Autodesk Inventor part; units mm, degrees
ref_plane "YZ Plane" through (0, 0, 0) normal (1, 0, 0) x (0, 1, 0)
ref_plane "XZ Plane" through (0, 0, 0) normal (0, 1, 0) x (-1, 0, 0)
ref_plane "XY Plane" through (0, 0, 0) normal (0, 0, 1) x (1, 0, 0)
sketch "Skizze1" plane through (0, 0, 0) normal (0, 0, 1) x (1, 0, 0)
  arc A0 (-7.910725, 24.207043) -> (-7.910891, 20.407043) centre (-6.063513, 22.306962) ccw
  line L0 (-7.910725, 24.207043) -> (-4.216135, 24.206882)
  arc A1 (-4.216301, 20.406882) -> (-4.216135, 24.206882) centre (-6.063513, 22.306962) ccw
  line L1 (-4.216301, 20.406882) -> (-7.910891, 20.407043)
  spline S0 degree 3 poles (4.168227, 35.189684) (1.190462, 36.459804) (-2.249662, 35.164227) (-6.254955, 34.158153) (-11.73606, 32.147863) (-17.267484, 27.437) (-17.397864, 22.280527) (-19.179409, 11.837341) (-24.204265, -4.219772) (-21.912215, -21.361857) (-15.72629, -32.136108) (-8.960071, -34.873142) (-7.734356, -35.206805) knots 0 0 0 0 0.05534958 0.07652777 0.21178189 0.29554676 0.38296386 0.43292215 0.75488434 0.81234043 0.96723776 1 1 1 1
  spline S1 degree 3 poles (-7.734356, -35.206805) (-2.439109, -36.648242) (4.93418, -35.14496) (14.388893, -31.364077) (20.220621, -28.276552) (23.084745, -23.179223) (23.280953, -18.995872) (17.306215, -16.499664) (13.73981, -19.293705) (6.907357, -22.933236) (-1.198572, -27.162074) (-10.305482, -22.9326) (-14.035245, -10.40017) (-9.459871, -0.926027) (-6.833349, 0.315314) (-5.918232, 2.05884) (-5.936684, 4.17913) (-8.288714, 5.230646) (-8.364147, 10.437319) (-1.010592, 14.125066) (4.082108, 20.05073) (3.063503, 26.302613) (2.949283, 28.613576) (3.78883, 29.833993) (5.577793, 31.092404) (6.613193, 32.774527) (5.245759, 34.708646) (4.265654, 35.148112) (4.168227, 35.189684) knots 0 0 0 0 0.1415298 0.17035016 0.24598676 0.2589199 0.29022703 0.32626485 0.37223258 0.38897966 0.48209608 0.50825566 0.62441589 0.64741797 0.71527435 0.72606992 0.74689162 0.80172241 0.81188461 0.84851364 0.9163561 0.94337427 0.94821885 0.96295932 0.96650966 0.98187972 0.99818797 1 1 1 1
  line L2 (-4.216301, 20.406882) -> (-7.910891, 20.407043)
  arc A2 (-4.216301, 20.406882) -> (-4.216135, 24.206882) centre (-6.063513, 22.306962) ccw
  line L3 (-7.910725, 24.207043) -> (-4.216135, 24.206882)
  arc A3 (-7.910725, 24.207043) -> (-7.910891, 20.407043) centre (-6.063513, 22.306962) ccw
  line L4 (-22.994876, 35.829551) -> (22.994876, 35.829551) construction
  line L5 (22.994876, 35.829551) -> (22.994876, -35.829551) construction
  line L6 (22.994876, -35.829551) -> (-22.994876, -35.829551) construction
  line L7 (-22.994876, -35.829551) -> (-22.994876, 35.829551) construction
  line L8 (-22.994876, 35.829551) -> (22.994876, -35.829551) construction
  line L9 (-22.994876, -35.829551) -> (22.994876, 35.829551) construction
  circle A4 centre (3.874552, -36.279551) radius 1.25 construction
  line L10 (1.214575, -35.829551) -> (11.587679, -35.829551) construction
  line L11 (3.874552, -36.279551) -> (3.874552, -35.029551) construction
  circle A5 centre (4.795469, 36.279551) radius 1.25 construction
  line L12 (4.795469, 36.279551) -> (4.795469, 35.029551) construction
  line L13 (3.124047, 35.829551) -> (12.547009, 35.829551) construction
  point P0 (0, 0)
  point P1 (0, 0)
  point P2 (0, 0)
  dimension "d88" = 2.5
  dimension "d91" = 2.5
  dimension "d89" = 0.8
  dimension "d92" = 0.8
sketch "Skizze9" plane through (0, 0, 0) normal (0, 0, 1) x (1, 0, 0)
  line L0 (-30, 46) -> (30, 46)
  line L1 (30, 46) -> (30, -46)
  line L2 (30, -46) -> (-30, -46)
  line L3 (-30, 46) -> (30, -46) construction
  line L4 (30, 46) -> (-30, -46) construction
  spline S0 degree 3 poles (4.168227, 35.189684) (1.190462, 36.459804) (-2.249662, 35.164227) (-6.254955, 34.158153) (-11.73606, 32.147863) (-17.267484, 27.437) (-17.397864, 22.280527) (-19.179409, 11.837341) (-24.204265, -4.219772) (-21.912215, -21.361857) (-15.72629, -32.136108) (-8.960071, -34.873142) (-7.734356, -35.206805) knots 0 0 0 0 0.05534958 0.07652777 0.21178189 0.29554676 0.38296386 0.43292215 0.75488434 0.81234043 0.96723776 1 1 1 1
  spline S1 degree 3 poles (-7.734356, -35.206805) (-2.439109, -36.648242) (4.93418, -35.14496) (14.388893, -31.364077) (20.220621, -28.276552) (23.084745, -23.179223) (23.280953, -18.995872) (17.306215, -16.499664) (13.73981, -19.293705) (6.907357, -22.933236) (-1.198572, -27.162074) (-10.305482, -22.9326) (-14.035245, -10.40017) (-9.459871, -0.926027) (-6.833349, 0.315314) (-5.918232, 2.05884) (-5.936684, 4.17913) (-8.288714, 5.230646) (-8.364147, 10.437319) (-1.010592, 14.125066) (4.082108, 20.05073) (3.063503, 26.302613) (2.949283, 28.613576) (3.78883, 29.833993) (5.577793, 31.092404) (6.613193, 32.774527) (5.245759, 34.708646) (4.265654, 35.148112) (4.168227, 35.189684) knots 0 0 0 0 0.1415298 0.17035016 0.24598676 0.2589199 0.29022703 0.32626485 0.37223258 0.38897966 0.48209608 0.50825566 0.62441589 0.64741797 0.71527435 0.72606992 0.74689162 0.80172241 0.81188461 0.84851364 0.9163561 0.94337427 0.94821885 0.96295932 0.96650966 0.98187972 0.99818797 1 1 1 1
  circle A0 centre (-3.5, -23.6754) radius 2
  circle A1 centre (5.000912, 27.85018) radius 2
  circle A2 centre (-6.3, 8.375362) radius 2
  line L5 (-30, -35.829553) -> (30, -35.829553)
  line L6 (-30, -46) -> (-30, 46)
  line L7 (-30, 35.829552) -> (30, 35.829552)
  point P0 (0, 0)
  point P1 (-2.781906, -35.829553)
  point P2 (1.073951, 35.829552)
  dimension "Laenge_aussen" = 105
  dimension "d68" = 60
  dimension "d69" = 92
  dimension "d180" = 4
  dimension "d182" = 4
  dimension "d183" = 4
  dimension "d184" = 33.5
  dimension "d186" = 24.99909
  dimension "d221" = 36.3
extrude "Extrusion3" add sketch "Skizze9" along normal blind 5 contours L0 L1 L7 L6 | L5 L1 L2 L6
sketch "Skizze11" plane through (0, 0, 0) normal (0, 0, -1) x (-1, 0, 0)
  line L0 (30, -46) -> (-30, -46)
  line L1 (30, 46) -> (30, -46)
  line L2 (-30, -46) -> (30, -46)
  line L3 (30, -46) -> (30, 46)
  line L4 (30, 46) -> (-30, 46)
  line L5 (-30, 46) -> (-30, -46)
  point P0 (0, 0)
extrude "Extrusion4" add sketch "Skizze11" along normal blind 1.5
chamfer "Fasen2" distance 0.5 angle 45 2 edges at (0, -35.8296, 5) (0, 35.8296, 5)
sketch "Skizze15" plane through (-30, 46, 5) normal (0, 1, 0) x (1, 0, 0)
  line L0 (60, 0) -> (0, 0)
  line L1 (0, 6.5) -> (60, 6.5)
  line L2 (60, 0) -> (0, 0)
  line L3 (0, 0) -> (0, 6.5)
  line L4 (0, 6.5) -> (60, 6.5)
  line L5 (60, 6.5) -> (60, 0)
  point P0 (30, 5)
extrude "Extrusion6" add sketch "Skizze15" along normal blind 4
sketch "Skizze16" plane through (-30, -46, 5) normal (0, -1, 0) x (1, 0, 0)
  line L0 (0, -6.5) -> (0, 0)
  line L1 (60, -6.5) -> (0, -6.5)
  line L2 (0, 0) -> (60, 0)
  line L3 (60, 0) -> (60, -6.5)
  line L4 (60, -6.5) -> (0, -6.5)
  line L5 (0, -6.5) -> (0, 0)
  point P0 (30, -5)
extrude "Extrusion7" add sketch "Skizze16" along normal blind 4
sketch "Skizze17" plane through (0, 0, -1.5) normal (0, 0, -1) x (-1, 0, 0)
  line L0 (30, 50) -> (30, -50)
  line L1 (-30, 50) -> (30, 50)
  line L2 (-30, -50) -> (-30, 50)
  line L3 (30, -50) -> (-30, -50)
  point P0 (0, 0)
extrude "Extrusion8" add sketch "Skizze17" along normal blind 3.5
chamfer "Fasen4" distance 0.5 angle 45 2 edges at (0, 50, 5) (0, -50, 5)
sketch "Skizze20" plane through (0, 0, 0) normal (0, 0, 1) x (1, 0, 0)
  line L0 (-30, -50) -> (30, -50)
  line L1 (30, 35.829552) -> (30, -35.829553)
  point P0 (0, 0)
  point P1 (-30, -46.5)
  point P2 (0, 0)
hole "Bohrung10" at (0, 0, 0) direction (0, 0, -1) diameter 5.5 end through all countersink diameter 11.5 countersink angle 90
sketch "Skizze21" plane through (-30, -50, 5) normal (0, -1, 0) x (1, 0, 0)
  line L0 (60, -10) -> (0, -10)
  line L1 (60, 0) -> (0, 0)
  line L2 (60, -0.5) -> (60, -10)
  line L3 (0, -0.5) -> (0, -10)
  point P0 (30, -5)
  point P1 (15, -5)
  point P2 (45, -5)
  point P3 (60, -5.25)
  dimension "d161" = 10
  dimension "d163" = 60
  dimension "d164" = 15
  dimension "d165" = 15
  dimension "d179" = 5
hole "Bohrung11" at (15, -50, 0) at (-15, -50, 0) direction (0, 1, 0) diameter 4.134 depth 6 tip angle 118
chamfer "Fasen5" distance 0.5 angle 45 2 edges at (-15, -50, 2.067) (15, -50, 2.067)
mirror "Spiegeln4" about plane through (0, 0, 0) normal (0, 1, 0) of "Bohrung11"
chamfer "Fasen6" distance 0.5 angle 45 2 edges at (15, 50, 2.067) (-15, 50, 2.067)
sketch "Skizze22" plane through (0, 0, 0) normal (0, 0, 1) x (1, 0, 0)
  circle A0 centre (-8.52675, -36.279553) radius 1.25 construction
  line L0 (30, -35.829553) -> (-30, -35.829553) construction
  line L1 (-19.029206, -35.029553) -> (-13.234121, -35.029553) construction
  spline S0 degree 3 poles (4.168227, 35.189684) (1.190462, 36.459804) (-2.249662, 35.164227) (-6.254955, 34.158153) (-11.73606, 32.147863) (-17.267484, 27.437) (-17.397864, 22.280527) (-19.179409, 11.837341) (-24.204265, -4.219772) (-21.912215, -21.361857) (-15.72629, -32.136108) (-8.960071, -34.873142) (-7.734356, -35.206805) knots 0 0 0 0 0.05534958 0.07652777 0.21178189 0.29554676 0.38296386 0.43292215 0.75488434 0.81234043 0.96723776 1 1 1 1 construction
  circle A1 centre (-3.073907, 36.279552) radius 1.25 construction
  line L2 (-18.70543, 35.029552) -> (-14.396256, 35.029552) construction
  line L3 (-30, 35.829552) -> (30, 35.829552) construction
  point P0 (0, 0)
  dimension "d188" = 2.5
  dimension "d189" = 0.8
  dimension "d190" = 2.5
  dimension "d191" = 0.8
sketch "Skizze23" plane through (-30, -35.829553, 0) normal (0, 1, 0) x (1, 0, 0)
  line L0 (20.22325, 0) -> (22.72325, 0) construction
  line L1 (0, -5) -> (60, -5)
  line L2 (60, -4.5) -> (0, -4.5)
  line L3 (60, 0) -> (0, 0)
  point P0 (30, 0)
  point P1 (21.47325, -2.25)
  point P2 (21.47325, 0)
  dimension "d218" = 4.5
  dimension "d219" = 2.25
hole "Bohrung12" at (-8.52675, -35.829553, 2.25) direction (0, -1, 0) diameter 3.242 end through all
chamfer "Fasen7" distance 0.5 angle 45 2 edges at (-8.5267, -35.8296, 0.629) (-8.5267, -50, 0.629)
sketch "Skizze24" plane through (-30, 35.829552, 0) normal (0, -1, 0) x (1, 0, 0)
  line L0 (28.176093, 0) -> (25.676093, 0) construction
  line L1 (60, 5) -> (0, 5)
  line L2 (0, 0) -> (60, 0)
  line L3 (0, 4.5) -> (60, 4.5)
  point P0 (30, 0)
  point P1 (26.926093, 2.25)
  point P2 (26.926093, 0)
  dimension "d205" = 2.25
  dimension "d220" = 4.5
hole "Bohrung13" at (-3.073907, 35.829552, 2.25) direction (0, 1, 0) diameter 3.242 end through all
chamfer "Fasen8" distance 0.5 angle 45 2 edges at (-3.0739, 35.8296, 3.871) (-3.0739, 50, 3.871)
extrude "Extrusion10" cut sketch "Skizze9" against normal blind 3 contours A0 | A2 | A1
equation "\"d91\" = Kugeldurchmesser"
equation "\"d89\" = Kugelhoehe"
equation "\"d92\" = Kugelhoehe"
equation "\"Laenge_aussen\" = Laenge_innen + 2 * Wanddicke"
equation "\"d68\" = Breite_innen"
equation "\"d191\" = d189"
equation "\"Breite_innen\" = 60"
equation "\"Laenge_innen\" = 85"
equation "\"Absatz\" = 2"
equation "\"Kugeldurchmesser\" = 2.5"
equation "\"Kugelhoehe\" = 0.8"
equation "\"Anbindung_Kolben\" = 15"
properties part number "TS_V1_Fallmagazin_Wandung_int"
Geometry: final body of the model. Coordinates: model frame, mm. A direction names the side the tool comes from. Round coordinates to 2 decimals unless told otherwise and drop trailing zeros. Loops run counter-clockwise (first coordinate to the right, second up) from the corner with the lowest first, then second, coordinate; pieces in that order, holes last. Notation, with made-up numbers: M -21,54 L -1,54 A16 ccw -1,65 Z; hole C -13,2.25 d5. An arc over 180 degrees is marked long. One line per question, with ' | ' between items.
(1) Cut plane C-C on x = 19.5. Return the cut outline in (y, z), plus the area to 3 significant figures.
Check result:
outline: M -50,-5 L 50,-5 L 50,4.5 L 49.5,5 L 36.33,5 L 35.83,4.5 L 35.83,0 L -35.83,0 L -35.83,4.5 L -36.33,5 L -49.5,5 L -50,4.5 Z | area: 641 mm2
(2) Contact query for flat-ended pins moving along their axis: P1, Ø5, axis at x = 5, y = 27.85, coming from the +Z side; P2, Ø3.5, axis at x = -15, z = 0, coming from the -Y side; P3, Ø2.5, axis at x = -15, z = 0, coming from the +Y side; P4, Ø5, axis at x = 0, y = 0, coming from the +Z side. Output: stop coordinate, or through.
Check result:
P1: stops at z = 0 | P2: stops at y = -43.81 | P3: stops at y = 43.51 | P4: passes through
(3) Access query for faces 1 (the cylindrical face through (-12.95, 46.71, 0.27)), 2 (the flat face through (0, -50, 0)), 3 (the flat face through (0, -35.83, 2)), 4 (the cylindrical face through (-5.22, 10.06, -1.48)), 5 (the flat face through (0, 43, 5)). Directions: +Z, -Z, +X, -X, +Y, -Y. A direction counts if a zero-diameter tool reaches every point of the face in a straight line with its end or side. Return the directions, or none.
Check result:
face 1: +Y | face 2: +Z, -Z, +X, -X, -Y | face 3: +Z, +X, -X | face 4: +Z | face 5: +Z, +X, -X, +Y, -Y
(4) Cut plane A-A on x = 0. Return the cut outline in (y, z).
Check result:
outline: M -50,-5 L -2.75,-5 L -2.75,-3 L -5.75,0 L -35.83,0 L -35.83,4.5 L -36.33,5 L -49.5,5 L -50,4.5 Z; M 2.75,-5 L 50,-5 L 50,4.5 L 49.5,5 L 36.33,5 L 35.83,4.5 L 35.83,0 L 5.75,0 L 2.75,-3 Z
(5) Pull-direction query (Z, two-part tool) for faces 6 (the cylindrical face through (2.685, 0.596, -4.014)), 7 (the flat face through (7, 1, 0)), 8 (the cylindrical face through (12.95, -46.71, 0.27)), 9 (the cylindrical face through (-16.743, -46.712, -1.111)); classes: +Z half, -Z half, draft (parallel to the pull), parting line (faces both ways), or undercut.
Check result:
face 6: draft | face 7: +Z half | face 8: undercut | face 9: undercut
(6) Cut plane B-B on y = 0. Return the cut outline in (x, z).
Check result:
outline: M -30,-5 L -2.75,-5 L -2.75,-3 L -5.75,0 L -30,0 Z; M 2.75,-5 L 30,-5 L 30,0 L 5.75,0 L 2.75,-3 Z
(7) Material intervals for line 1 along X through (y, z) = (-47, 0); line 2 along Y through (x, z) = (4, -1); line 3 along Y through (x, z) = (23.5, 4.25), sorted ascending. Write a range as from..to.
Check result:
line 1: x = -30..-17.07, -12.93..12.93, 17.07..30 | line 2: y = -50..-2.56, 2.56..26.12, 29.58..50 | line 3: y = -50..-35.83, 35.83..50
